from build123d import *

# Parameters (mm, degrees)
SKETCH_R   = 5.175
SKETCH_R_2 = 36.1
PAD_DEPTH  = 20


with BuildPart() as chamfer_cutout_right:
    # Sketch002 → Revolution (revolve)
    with BuildSketch(Plane.YZ):
        with BuildLine():
            Line((36.1, 15.427249), (39.9, 15.427249))
            ThreePointArc((39.9, 15.427249), (48.804267, 7.330048), (58.35, 0))
            Line((58.35, 0), (58.35, -5))
            Line((58.35, -5), (36.1, -5))
            Line((36.1, -5), (36.1, 15.427249))
        make_face()
    revolve(axis=Axis((0, 0, 0), (0, 0, 1)))


with BuildPart() as spacer_right:
    # Sketch → Pad (new body)
    with BuildSketch(Plane.XY):
        with BuildLine():
            ThreePointArc((-15.484484, 45.433806), (-31.397174, 49.18272), (-34.694729, 33.170405))
            Line((-28.839993, 27.572899), (-34.694729, 33.170405))
            ThreePointArc((-28.839993, 27.572899), (0, -39.9), (28.839993, 27.572899))
            Line((28.839993, 27.572899), (34.694729, 33.170405))
            ThreePointArc((34.694729, 33.170405), (31.397174, 49.18272), (15.484484, 45.433806))
            ThreePointArc((15.484484, 45.433806), (0, 48), (-15.484484, 45.433806))
        make_face()
        with Locations((-27.375, 42.882106)):
            Circle(SKETCH_R, mode=Mode.SUBTRACT)
        with Locations((27.375, 42.882106)):
            Circle(SKETCH_R, mode=Mode.SUBTRACT)
        Circle(SKETCH_R_2, mode=Mode.SUBTRACT)
    extrude(amount=PAD_DEPTH)

    # Cut: cut chamfer_cutout_right
    add(chamfer_cutout_right.part, mode=Mode.SUBTRACT)


solid = spacer_right.part
Check sheet for the modelled part. Datum: model origin and axes. Units: mm. A direction names the side the tool comes from. Coordinates: 2 decimals unless noted, no trailing zeros. Loops run counter-clockwise (first coordinate to the right, second up) from the corner with the lowest first, then second, coordinate; pieces in that order, holes last. Notation, with made-up numbers: (74, -19) -> (131, -19) arc R16 cw to (131, 11) -> close; hole circle Ø9 at (-15.5, -32.75). An arc over 180 degrees is marked (long way). Write item = value, one per line. Start each with the question number.
1. Material ranges on line 1 (Y direction, x = 0, z = 18.8); line 2 (X direction, y = 44, z = 16.25); line 3 (Y direction, x = -31, z = 16.75) (3 decimals), recorded low to high.
2. Section check A-A on y = 0. Record the cut outline in (x, z).
3. Draft check along Y on faces 1 (the cylindrical face through (-1.3, -39.88, 17.68)), 2 (the flat face through (21, 30, 15.427)), 3 (the cylindrical face through (0, 48, 14)). Enter one of: released by +Y, released by -Y, zero draft, split by the parting line, or undercut.
4. Depth check by flat-ended pin: P1, Ø10, axis at x = 23, z = 5, coming from the +Y side; P2, Ø4, axis at x = -31.5, z = 2, coming from the +Y side; P3, Ø24, axis at x = -19.5, y = -15.5, coming from the -Z side; P4, Ø6, axis at y = 15, z = 14.5, coming from the -X side. Enter the tip coordinate at first touch or a pass-through.
5. Tool access check on faces 4 (the flat face through (-32.377, 30.954, 15.252)), 5 (the flat face through (32.377, 30.954, 15.252)), 6 (the cylindrical face through (31.611, 49.043, 12.081)). Record the directions out of +Z, -Z, +X, -X, +Y, -Y that give a thin tool (end or side, any length) a straight path to the whole face; none if there is none.
6. Section check C-C on x = 23.5. Give the number of separate pieces and of enclosed holes in the cut face, then the cut area to 3 significant figures.
7. Section check B-B on y = 14. Record the cut outline in (x, z).
Responses:
q1.line_1 = -39.9 to -36.1, 36.1 to 48
q1.line_2 = -35.77 to -32.43, -22.32 to 22.32, 32.43 to 35.77
q1.line_3 = -25.12 to -18.499, 18.499 to 25.12, 29.638 to 39.189, 46.575 to 49.425
q2.outline = (-39.9, 15.43) -> (-36.1, 15.43) -> (-36.1, 20) -> (-39.9, 20) -> close; (36.1, 15.43) -> (39.9, 15.43) -> (39.9, 20) -> (36.1, 20) -> close
q3.face_1 = undercut
q3.face_2 = zero draft
q3.face_3 = released by +Y
q4.P1 = 50.97
q4.P2 = 50.16
q4.P3 = 15.43
q4.P4 = -38.01
q5.face_4 = +Z, -Z, -X
q5.face_5 = +Z, -Z, +X
q5.face_6 = +Z, -Z
q6.separate_pieces = 3
q6.enclosed_holes = 0
q6.area = 174 mm2
q7.outline = (-37.36, 15.43) -> (-33.27, 15.43) -> (-33.27, 20) -> (-37.36, 20) -> close; (33.27, 15.43) -> (37.36, 15.43) -> (37.36, 20) -> (33.27, 20) -> close
